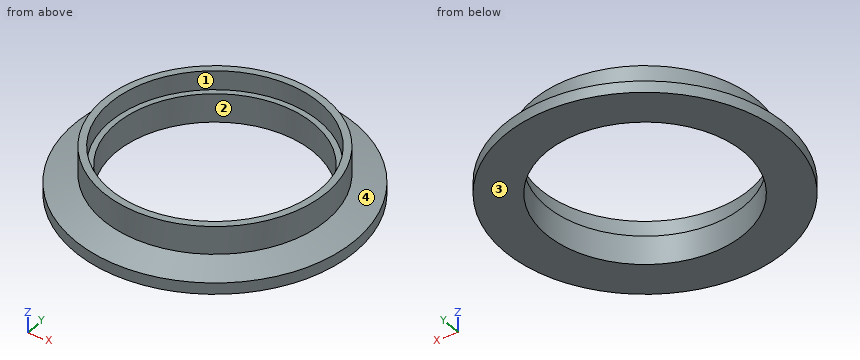
Autodesk Inventor part; units mm, degrees
ref_plane "YZ Plane" through (0, 0, 0) normal (1, 0, 0) x (0, 1, 0)
ref_plane "XZ Plane" through (0, 0, 0) normal (0, 1, 0) x (-1, 0, 0)
sketch "Sketch1" plane through (0, 0, 0) normal (0, 0, 1) x (1, 0, 0)
  circle A0 centre (0, 0) radius 37.465
  dimension "d0" = 74.93
extrude "Extrusion1" add sketch "Sketch1" along normal blind 12.7
sketch "Sketch3" plane through (0, 0, 12.7) normal (0, 0, 1) x (1, 0, 0)
  circle A0 centre (0, 0) radius 26.289
  dimension "d6" = 52.578
extrude "Extrusion3" cut sketch "Sketch3" against normal blind 2.54
sketch "Sketch4" plane through (0, 0, 0) normal (0, 0, -1) x (-1, 0, 0)
  circle A0 centre (0, 0) radius 26.416
  dimension "d9" = 52.832
extrude "Extrusion4" cut sketch "Sketch4" against normal blind 2.54
ref_plane "Work Plane1" through (0, 0, 12.7) normal (0, 0, 1) x (1, 0, 0)
ref_plane "Work Plane3" through (0, 0, 5.2324) normal (0, 0, 1) x (1, 0, 0)
ref_plane "Work Plane5" through (0, 0, 3.048) normal (0, 0, 1) x (1, 0, 0)
sketch "Sketch9" plane through (0, 0, 5.2324) normal (0, 0, 1) x (1, 0, 0)
  circle A0 centre (0, 0) radius 29.845
sketch "Sketch11" plane through (0, 0, 3.048) normal (0, 0, 1) x (1, 0, 0)
  circle A0 centre (0, 0) radius 29.845
  circle A1 centre (0, 0) radius 37.465
  dimension "d42" = 59.69
  dimension "d43" = 74.93
extrude "Extrusion7" cut sketch "Sketch11" along normal through all
loft "Loft5" add profiles "Sketch9" section 2 edges at (-37.465, 0, 3.048)
sketch "Sketch12" plane through (0, 0, 12.7) normal (0, 0, 1) x (1, 0, 0)
  circle A0 centre (0, 0) radius 27.94
  circle A1 centre (0, 0) radius 26.289
  dimension "d50" = 55.88
extrude "Extrusion8" cut sketch "Sketch12" against normal blind 5.08
sketch "Sketch2" plane through (0, 0, 12.7) normal (0, 0, 1) x (1, 0, 0)
  circle A0 centre (0, 0) radius 26.416
  dimension "d3" = 52.832
extrude "Extrusion2" cut sketch "Sketch2" against normal blind 50.8
properties part number "KF50tube_v3"
Geometry: final body of the model. Coordinates: model frame, mm. Face numbers are marked on the shaded views. Give positions to 0.01 mm unless a question says otherwise; leave off trailing zeros. Order: outer loops, then holes, each group sorted by start corner. A loop starts at its lowest first (then second) coordinate and runs counter-clockwise, first axis right, second up. Notation, with made-up numbers: (24.25, -20.5) -> (77.25, -20.5) arc R10 cw to (77.25, -16.5) -> close; hole circle Ø1 at (-38, -31.5). An arc over 180 degrees is marked (long way). Put each result on its own line as item: value.
Q1. Section B-B, the plane z = 8.75. Return loops of the section in (x, y) (3 decimals).
Here are the results:
outline: circle Ø59.69 at (0, 0); hole circle Ø55.88 at (0, 0)
Q2. Pin query (flat end, axial travel): pin 1 (3 mm diameter, centred on x = -24, z = 11, fed in from +Y); pin 2 (17 mm diameter, centred on x = 8.5, y = -11.5, fed in from +Z); pin 3 (10 mm diameter, centred on x = 28.5, y = -10.5, fed in from +Z); pin 4 (1.5 mm diameter, centred on x = -22, z = 9.5, fed in from +Y). Return the tip coordinate at first contact, or that it passes through.
Here are the results:
pin 1: stops at y = 19.61
pin 2: passes through
pin 3: stops at z = 12.7
pin 4: stops at y = 20.96
Q3. Draft query along X for the marked faces 1, 2, 3 and 4. Return one class per face: released by +X, released by -X, zero draft, split by the parting line, or undercut.
Here are the results:
face 1: undercut
face 2: undercut
face 3: zero draft
face 4: split by the parting line
Q4. Section A-A, the plane x = 0. Return loops of the section in (y, z) (3 decimals).
Here are the results:
outline: (-37.465, 0) -> (-26.416, 0) -> (-26.416, 7.62) -> (-27.94, 7.62) -> (-27.94, 12.7) -> (-29.845, 12.7) -> (-29.845, 5.232) -> (-37.465, 3.048) -> close; (26.416, 0) -> (37.465, 0) -> (37.465, 3.048) -> (29.845, 5.232) -> (29.845, 12.7) -> (27.94, 12.7) -> (27.94, 7.62) -> (26.416, 7.62) -> close
Q5. Material intervals for L1, parallel to Y at x = 0, z = 11.25 (3 decimals); L2, parallel to Y at x = -3, z = 9.75; L3, parallel to Z at x = -20, y = 18, sorted ascending.
Here are the results:
L1: y = -29.845 to -27.94, 27.94 to 29.845
L2: y = -29.69 to -27.78, 27.78 to 29.69
L3: z = 0 to 7.62
